```python
from build123d import *

# Parameters (mm, degrees)
SKETCH1_R           = 4
BOSS_EXTRUDE1_DEPTH = 10
BOSS_EXTRUDE2_START = 8
SKETCH2_R           = 4
BOSS_EXTRUDE2_DEPTH = 8
FILLET3_R           = 1


with BuildPart() as part:
    # Sketch1 → Boss-Extrude1 (new body)
    with BuildSketch(Plane(origin=(0, 0, 0), x_dir=(1, 0, 0), z_dir=(0, 1, 0))):
        with Locations(Location((0, 0, 0), (0, 0, 270))):
            Circle(SKETCH1_R)
    extrude(amount=BOSS_EXTRUDE1_DEPTH)

    # Sketch2 → Boss-Extrude2 (add)
    with BuildSketch(Plane.XZ.offset(BOSS_EXTRUDE2_START)):
        with Locations(Location((0, 0, 0), (0, 0, 270))):
            Circle(SKETCH2_R)
        with BuildLine():
            Line((-3.03407729, -0.5), (3.03407729, -0.5))
            ThreePointArc((3.03407729, -0.5), (0, -3.075), (-3.03407729, -0.5))
        make_face(mode=Mode.SUBTRACT)
        with BuildLine():
            Line((-3.03407729, 0.5), (3.03407729, 0.5))
            ThreePointArc((3.03407729, 0.5), (0, 3.075), (-3.03407729, 0.5))
        make_face(mode=Mode.SUBTRACT)
    extrude(amount=-BOSS_EXTRUDE2_DEPTH)

    # Fillet3
    fillet3_edges = [part.edges().sort_by_distance(p)[0] for p in [
        (0, 10, -4),
    ]]
    fillet(fillet3_edges, radius=FILLET3_R)


solid = part.part
```
Here's how the part is built. I have some questions about the finished solid (model axes, mm). A direction names the side the tool comes from. Coordinates: 2 decimals unless noted, no trailing zeros. Loops run counter-clockwise (first coordinate to the right, second up) from the corner with the lowest first, then second, coordinate; pieces in that order, holes last. Notation, with made-up numbers: (24.5, 10.25) - (77.5, 10.25) arc R9 cw to (77.5, 17.25) - close; hole circle Ø2 at (-28, -7). An arc over 180 degrees is marked (long way). Answer as CSV lines item,"result".
Q1. If we section it at A-A, the plane y = -2.75: Write out the boundary of the cut face in (x, z) (3 decimals), and give its area (3 significant figures).
Response:
outline,"circle Ø8 at (0, 0); hole (-3.034, -0.5) arc R3.075 ccw to (3.034, -0.5) - close; hole (-3.034, 0.5) - (3.034, 0.5) arc R3.075 ccw to start"
area,"26.7 mm2"
Q2. If we section it at C-C, the plane y = 6: Write out the boundary of the cut face in (x, z), and give its area (3 significant figures).
Response:
outline,"circle Ø8 at (0, 0)"
area,"50.3 mm2"
Q3. For faces 3 (the face through (0, 10, 0)), 4 (the face through (0, -4, -0.5)), which set-ups out of +Z, -Z, +X, -X, +Y, -Y let a thin tool reach every point of the face, with its end or its side?
Response:
face 3,"+Z, -Z, +X, -X, +Y"
face 4,"-Y"
Q4. We'd pull the mould along Z, two halves only. Please class faces 1 (the face through (0, -8, 0)), 2 (the face through (0, 0, -2)): pulls with the +Z half, pulls with the -Z half, needs draft (parallel to the pull), parting line crosses it, or undercut.
Response:
face 1,"needs draft"
face 2,"undercut"
Q5. For pin 1 (1.3 mm diameter, centred on x = 0, z = -2, fed in from -Y); pin 2 (2 mm diameter, centred on y = 7, z = -2, fed in from +X); pin 3 (1.5 mm diameter, centred on y = -0.5, z = -1, fed in from +X), each with a flat end and sliding along its axis, tell me the tip position at first contact or that it passes through.
Response:
pin 1,"y = 0"
pin 2,"x = 3.87"
pin 3,"x = 3.99"
Q6. If we section it at B-B, the plane x = 0: Write out the boundary of the cut face in (y, z) (3 decimals), and give its area (3 significant figures).
Response:
outline,"(-8, -4) - (9, -4) arc R1 ccw to (10, -3) - (10, 3) arc R1 ccw to (9, 4) - (-8, 4) - (-8, 3.075) - (0, 3.075) - (0, 0.5) - (-8, 0.5) - (-8, -0.5) - (0, -0.5) - (0, -3.075) - (-8, -3.075) - close"
area,"102 mm2"
Q7. If I drill on L1, parallel to Z at x = -0.25, y = -6.5; L2, parallel to Z at x = 1, y = -5; L3, parallel to X at y = -4.5, z = -1, over which ranges is the centre line in solid material (lowest first)? Write a range as [from, to].
Response:
L1,"[-3.99, -3.06], [-0.5, 0.5], [3.06, 3.99]"
L2,"[-3.87, -2.91], [-0.5, 0.5], [2.91, 3.87]"
L3,"[-3.87, -2.91], [2.91, 3.87]"
